Here's how the part is built. I have some questions about the finished solid (model axes, mm). Round coordinates to 2 decimals unless told otherwise and drop trailing zeros. Write each loop counter-clockwise with the first axis right and the second up, starting at its lowest first coordinate (ties: lowest second). Pieces come first, ordered by that corner, then holes. Notation, with made-up numbers: (-23, 67) - (-7, 67) arc R13 ccw to (-7, 71) - close; hole circle Ø4 at (12, 12.25). An arc over 180 degrees is marked (long way). Write item = value, one per line. Start each with the question number.
Item 1: Thinking about a two-plate mould opening in X: for faces 1 (the face through (11.097, 1.972, -110.698)), 2 (the face through (2.85, 2.03, -3.01)), 3 (the face through (60, 4, -59)), which applies, pulls with the +X half, pulls with the -X half, needs draft (parallel to the pull), parting line crosses it, or undercut?
Item 2: If we section it at A-A (x = 23.5): Please give me the cut outline in (y, z), and give its area (3 significant figures).
Item 3: If we section it at B-B (z = -96): Please give me the cut outline in (x, y), and give its area (3 significant figures).
Item 4: If I drill on line 1 along X through (y, z) = (3, -96); line 2 along X through (y, z) = (1.35, -8.5); line 3 along Z through (x, y) = (8, 2.85), over which ranges is the centre line in solid material (lowest first)? Write a range as [from, to].
```python
from build123d import *

# Parameters (mm, degrees)
SKETCH1_W           = 122
SKETCH1_H           = 117
SKETCH1_R           = 2.2
BOSS_EXTRUDE1_DEPTH = 4
FILLET1_R           = 10


with BuildPart() as part:
    # Sketch1 → Boss-Extrude1 (new body)
    with BuildSketch(Plane(origin=(0, 0, 0), x_dir=(1, 0, 0), z_dir=(0, 1, 0))):
        with Locations((61, 58.5)):
            Rectangle(SKETCH1_W, SKETCH1_H)
        with Locations(Location((111, 108.5, 0), (0, 0, 270))):
            Circle(SKETCH1_R, mode=Mode.SUBTRACT)
        with Locations(Location((11, 108.5, 0), (0, 0, 270))):
            Circle(SKETCH1_R, mode=Mode.SUBTRACT)
        with Locations(Location((11, 8.5, 0), (0, 0, 270))):
            Circle(SKETCH1_R, mode=Mode.SUBTRACT)
        with Locations(Location((111, 8.5, 0), (0, 0, 270))):
            Circle(SKETCH1_R, mode=Mode.SUBTRACT)
        with Locations(Location((98.5, 96, 0), (0, 0, 270))):
            Circle(SKETCH1_R, mode=Mode.SUBTRACT)
        with Locations(Location((23.5, 96, 0), (0, 0, 270))):
            Circle(SKETCH1_R, mode=Mode.SUBTRACT)
        with Locations(Location((23.5, 21, 0), (0, 0, 270))):
            Circle(SKETCH1_R, mode=Mode.SUBTRACT)
        with Locations(Location((98.5, 21, 0), (0, 0, 270))):
            Circle(SKETCH1_R, mode=Mode.SUBTRACT)
    extrude(amount=BOSS_EXTRUDE1_DEPTH)

    # Fillet1
    fillet1_edges = [part.edges().sort_by_distance(p)[0] for p in [
        (0, 2, -117),
        (122, 2, -117),
        (122, 2, 0),
        (0, 2, 0),
    ]]
    fillet(fillet1_edges, radius=FILLET1_R)


solid = part.part
```
Reply:
q1.face_1 = undercut
q1.face_2 = pulls with the -X half
q1.face_3 = needs draft
q2.outline = (0, -117) - (4, -117) - (4, -98.2) - (0, -98.2) - close; (0, -93.8) - (4, -93.8) - (4, -23.2) - (0, -23.2) - close; (0, -18.8) - (4, -18.8) - (4, 0) - (0, 0) - close
q2.area = 433 mm2
q3.outline = (0, 0) - (21.3, 0) - (21.3, 4) - (0, 4) - close; (25.7, 0) - (96.3, 0) - (96.3, 4) - (25.7, 4) - close; (100.7, 0) - (122, 0) - (122, 4) - (100.7, 4) - close
q3.area = 453 mm2
q4.line_1 = [0, 21.3], [25.7, 96.3], [100.7, 122]
q4.line_2 = [0.11, 8.8], [13.2, 108.8], [113.2, 121.89]
q4.line_3 = [-116.8, -0.2]
